Here's how the part is built. I have some questions about the finished solid (model axes, mm). A direction names the side the tool comes from. Coordinates: 2 decimals unless noted, no trailing zeros. Loops run counter-clockwise (first coordinate to the right, second up) from the corner with the lowest first, then second, coordinate; pieces in that order, holes last. Notation, with made-up numbers: (-14.75, -36.75) -> (1.25, -36.75) arc R18 ccw to (1.25, -5.75) -> close; hole circle Ø5 at (-7, 83.25). An arc over 180 degrees is marked (long way). Answer as a JSON object with one key per item and string values. Group by question number.
Q1. Thinking about a two-plate mould opening in Y: for faces 1 (the conical face through (2.237, 164.941, 10.074)), 2 (the cylindrical face through (-14.854, -12.622, 8.211)), 3 (the cylindrical face through (2.75, 80.14, 12.4)), which applies, released by +Y, released by -Y, zero draft, split by the parting line, or undercut?
Q2. On a 3-axis mill with a long thin cutter (end or side, diameter ignored), from which of +Z, -Z, +X, -X, +Y, -Y can I reach the whole of each face in a straight line? I mean faces 4 (the flat face through (0, 0, -13)), 5 (the flat face through (0, -6, -20.32)), 6 (the conical face through (9.842, 165.259, -3.1)). Say none if no direction works.
Q3. I need wall thicknesses on line 1 (Y direction, x = 11, z = -15.5); line 2 (Y direction, x = 9.5, z = 6.5); line 3 (Y direction, x = 17, z = 6.5). Which ranges of each line are inside material? Lowest first, please.
Q4. I want a section at B-B on y = 171.5. Write out the boundary of the cut face in (x, z), then the cut area to 3 significant figures.
Q5. I'm going to push flat-ended pins straight in: pin 1 (2 mm diameter, centred on x = 12.5, y = 142, fed in from -Z); pin 2 (10 mm diameter, centred on y = 75.5, z = 8.5, fed in from -X); pin 3 (1 mm diameter, centred on x = 1.5, y = 26.5, fed in from -Z). Where does each tip first touch, or does it pass through?
Autodesk Inventor part; units mm, degrees
ref_plane "YZ Plane" through (0, 0, 0) normal (1, 0, 0) x (0, 1, 0)
ref_plane "XZ Plane" through (0, 0, 0) normal (0, 1, 0) x (-1, 0, 0)
ref_plane "XY Plane" through (0, 0, 0) normal (0, 0, 1) x (1, 0, 0)
sketch "Sketch1" plane through (0, 0, 0) normal (0, 1, 0) x (-1, 0, 0)
  circle A0 centre (0, 0) radius 12.7
  dimension "d0" = 25.4
extrude "Extrusion1" add sketch "Sketch1" along normal blind 165.1
sketch "Sketch2" plane through (0, 165.1, 0) normal (0, 1, 0) x (1, 0, 0)
  circle A0 centre (0, 0) radius 12.7
chamfer "Chamfer1" distance 2.54 angle 45 1 edges at (12.7, 165.1, 0)
extrude "Extrusion2" add sketch "Sketch2" along normal blind 76.2
thread "Thread2"
chamfer "Chamfer2" distance 2.54 angle 45 1 edges at (-12.7, 165.1, 0)
sketch "Sketch3" plane through (0, 0, 0) normal (0, -1, 0) x (1, 0, 0)
  line L0 (0, 20.32) -> (0, -20.32) construction
  line L1 (0, -20.32) -> (11.43, -20.32) construction
  line L2 (11.43, -20.32) -> (-11.43, -20.32)
  line L3 (-11.43, -20.32) -> (-22.86, -0.5227)
  line L4 (-22.86, -0.5227) -> (-11.43, 19.2747)
  line L5 (-11.43, 19.2747) -> (11.43, 19.2747)
  line L6 (11.43, 19.2747) -> (22.86, -0.5227)
  line L7 (22.86, -0.5227) -> (11.43, -20.32)
  point P0 (0, 0)
  dimension "d18" = 20.32
  dimension "d19" = 40.64
  dimension "d20" = 11.43
  dimension "d21" = 22.86
  dimension "d22" = 22.86
  dimension "d23" = 120
  dimension "d24" = 22.86
  dimension "d25" = 22.86
  dimension "d26" = 120
extrude "Extrusion3" add sketch "Sketch3" along normal blind 12.7
chamfer "Chamfer3" distance 2.54 angle 45 6 edges at (0, -12.7, -20.32) (-17.145, -12.7, -10.4213) (-17.145, -12.7, 9.376) (0, -12.7, 19.2747) (17.145, -12.7, 9.376) (17.145, -12.7, -10.4213)
fillet "Fillet1" radius 1 12 edges at (-10.6968, -11.43, -19.05) (10.6968, -11.43, -19.05) (21.3935, -11.43, -0.5227) (10.6968, -11.43, 18.0047) (-10.6968, -11.43, 18.0047) (-21.3935, -11.43, -0.5227) (-14.9453, -12.7, -9.1513) (-14.9453, -12.7, 8.106) (0, -12.7, 16.7347) (14.9453, -12.7, 8.106) (14.9453, -12.7, -9.1513) (0, -12.7, -17.78)
fillet "Fillet2" radius 1 12 edges at (11.43, -5.0343, -20.32) (22.86, -5.0343, -0.5227) (11.43, -5.0343, 19.2747) (-11.43, -5.0343, 19.2747) (-22.86, -5.0343, -0.5227) (-11.43, -5.0343, -20.32) (-17.145, 0, 9.376) (-17.145, 0, -10.4213) (0, 0, 19.2747) (17.145, 0, 9.376) (17.145, 0, -10.4213) (0, 0, -20.32)
properties part number "CIM Mount Bolt" material "Aluminum 6061-AHC"
Result set:
{
 "1": {"face 1": "undercut", "face 2": "released by -Y", "face 3": "zero draft"},
 "2": {"face 4": "+Y", "face 5": "-Z, +X, -X, +Y, -Y", "face 6": "none"},
 "3": {"line 1": "y = -12.69 to 0", "line 2": "y = -12.7 to 163.75, 166.45 to 241.3", "line 3": "y = -11.72 to 0"},
 "4": {"outline": "circle Ø25.4 at (0, 0)", "area": "507 mm²"},
 "5": {"pin 1": "stops at z = -5.39", "pin 2": "stops at x = -12.21", "pin 3": "stops at z = -12.66"}
}
